Part model, mm, in its own coordinate system. Face numbers are marked on the shaded views. A direction names the side the tool comes from. Round coordinates to 2 decimals unless told otherwise and drop trailing zeros. Order: outer loops, then holes, each group sorted by start corner. A loop starts at its lowest first (then second) coordinate and runs counter-clockwise, first axis right, second up. Notation, with made-up numbers: (76, 12.5) - (112, 12.5) arc R17 cw to (112, 26.5) - close; hole circle Ø10 at (46, 76.5). An arc over 180 degrees is marked (long way). Return JSON: item names as keys, results as strings. Group by question number.
Item 1: Saw through at B-B on x = 1.2. List the corners of the cut face in (y, z).
Item 2: Probe probe 1 along X at (y, z) = (0.75, -1); probe 2 along Z at (x, y) = (2.85, 1.1). List the from-to ranges inside material, lowest first.
Item 3: Tool access for the marked faces 1 and 2: list every direction of +Z, -Z, +X, -X, +Y, -Y with a clear straight run to the whole face (end or side of a thin tool).
Item 4: Two-plate mould, pull along Z, no slides. Class the marked faces 3, 4 and 5: released by +Z, released by -Z, zero draft, split by the parting line, or undercut.
Item 5: Saw through at A-A on y = 3.9. List the corners of the cut face in (x, z).
Item 6: Saw through at C-C on z = -5.25. List the corners of the cut face in (x, y), and give its area (3 significant figures).
```python
from build123d import *

# Parameters (mm, degrees)
CROQUIS1_W              = 4.39
CROQUIS1_H              = 6.1
SALIENTE_EXTRUIR1_DEPTH = 4.65
CROQUIS3_W              = 1.4
CROQUIS3_H              = 4.5
CORTAR_EXTRUIR1_DEPTH   = 9.837680691
CROQUIS4_R              = 0.143820832
CORTAR_EXTRUIR2_DEPTH   = 0.25


with BuildPart() as part:
    # Croquis1 → Saliente-Extruir1 (new body)
    with BuildSketch(Plane(origin=(0, 0, 0), x_dir=(1, 0, 0), z_dir=(0, 1, 0))):
        with Locations((2.195, 3.05)):
            Rectangle(CROQUIS1_W, CROQUIS1_H)
    extrude(amount=SALIENTE_EXTRUIR1_DEPTH)

    # Croquis3 → Cortar-Extruir1 (cut, through all)
    with BuildSketch(Plane(origin=(0, 4.65, 0), x_dir=(1, 0, 0), z_dir=(0, 1, 0))):
        with Locations((1.14, 3.077612144)):
            Rectangle(CROQUIS3_W, CROQUIS3_H)
        with Locations((3.256764551, 3.077612144)):
            Rectangle(CROQUIS3_W, CROQUIS3_H)
    extrude(amount=-CORTAR_EXTRUIR1_DEPTH, mode=Mode.SUBTRACT)

    # Croquis4 → Cortar-Extruir2 (cut)
    with BuildSketch(Plane(origin=(0, 4.65, 0), x_dir=(1, 0, 0), z_dir=(0, 1, 0))):
        with Locations(Location((0.353367476, 5.755686139, 0), (0, 0, 270))):
            Circle(CROQUIS4_R)
    extrude(amount=-CORTAR_EXTRUIR2_DEPTH, mode=Mode.SUBTRACT)


solid = part.part
```
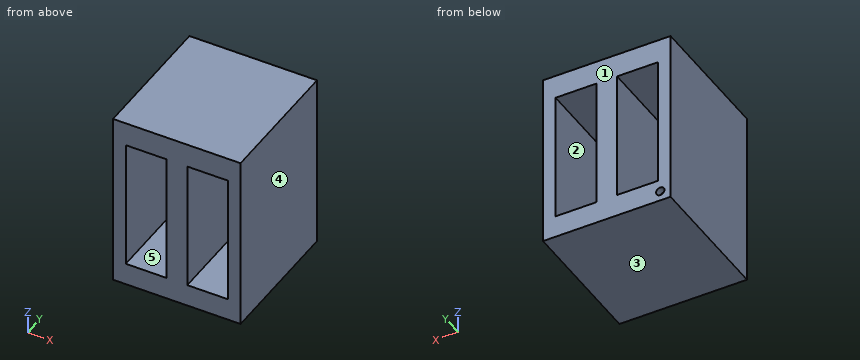
Filled in:
{
 "1": {"outline": "(0, -6.1) - (4.65, -6.1) - (4.65, -5.33) - (0, -5.33) - close; (0, -0.83) - (4.65, -0.83) - (4.65, 0) - (0, 0) - close"},
 "2": {"probe 1": "x = 0 to 0.44, 1.84 to 2.56, 3.96 to 4.39", "probe 2": "z = -6.1 to -5.33, -0.83 to 0"},
 "3": {"face 1": "+Z, -Z, +X, -X, +Y", "face 2": "+Y, -Y"},
 "4": {"face 3": "released by -Z", "face 4": "zero draft", "face 5": "undercut"},
 "5": {"outline": "(0, -6.1) - (4.39, -6.1) - (4.39, 0) - (0, 0) - close; hole (0.44, -5.33) - (1.84, -5.33) - (1.84, -0.83) - (0.44, -0.83) - close; hole (2.56, -5.33) - (3.96, -5.33) - (3.96, -0.83) - (2.56, -0.83) - close"},
 "6": {"outline": "(0, 0) - (0.44, 0) - (0.44, 4.65) - (0, 4.65) - close; (1.84, 0) - (2.56, 0) - (2.56, 4.65) - (1.84, 4.65) - close; (3.96, 0) - (4.39, 0) - (4.39, 4.65) - (3.96, 4.65) - close", "area": "7.39 mm^2"}
}
